Could you check a few things on this model? Use its own coordinates, in mm. Face numbers are marked on the shaded views. A direction names the side the tool comes from. Coordinates: 2 decimals unless noted, no trailing zeros. Write each loop counter-clockwise with the first axis right and the second up, starting at its lowest first coordinate (ties: lowest second). Pieces come first, ordered by that corner, then holes. Notation, with made-up numbers: M 77.5,-31 L 112.5,-31 A17 cw 112.5,-21 Z; hole C 11.5,28 d7. An arc over 180 degrees is marked long. Write item = value, one per line.
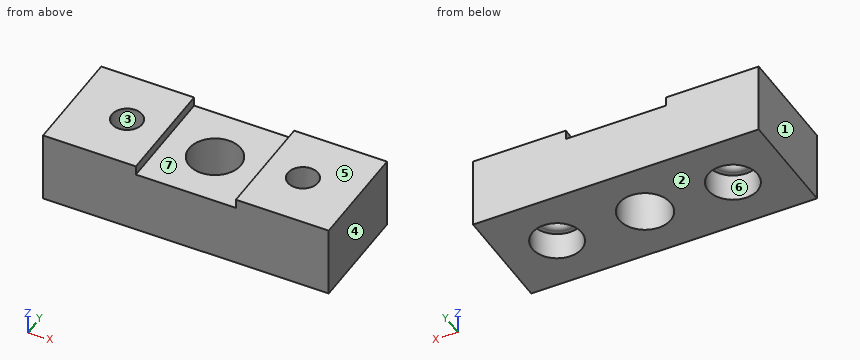
```python
from build123d import *

# Parameters (mm, degrees)
SKETCH_1_W          = 52
SKETCH_1_H          = 20
SKETCH_1_R          = 2.75
SKETCH_1_R_2        = 4.7
EXTRUDE_1_DEPTH     = 13
SKETCH_2_R          = 4.5
CUT_EXTRUDE_1_DEPTH = 5
SKETCH_3_W          = 18.2
SKETCH_3_H          = 20
CUT_EXTRUDE_2_DEPTH = 1.7
FILLET_1_R          = 1


with BuildPart() as part:
    # 草图1 → 凸台-拉伸1 (new body)
    with BuildSketch(Plane.XY):
        Rectangle(SKETCH_1_W, SKETCH_1_H)
        with Locations(Location((-16, 0, 0), (0, 0, 180))):
            Circle(SKETCH_1_R, mode=Mode.SUBTRACT)
        with Locations(Location((16, 0, 0), (0, 0, 180))):
            Circle(SKETCH_1_R, mode=Mode.SUBTRACT)
        with Locations(Location((0, 0, 0), (0, 0, 180))):
            Circle(SKETCH_1_R_2, mode=Mode.SUBTRACT)
    extrude(amount=EXTRUDE_1_DEPTH)

    # 草图2 → 切除-拉伸1 (cut)
    with BuildSketch(Plane(origin=(0, 0, 0), x_dir=(-1, 0, 0), z_dir=(0, 0, -1))):
        with Locations((-16, 0)):
            Circle(SKETCH_2_R)
        with Locations((16, 0)):
            Circle(SKETCH_2_R)
    extrude(amount=-CUT_EXTRUDE_1_DEPTH, mode=Mode.SUBTRACT)

    # 草图3 → 切除-拉伸2 (cut)
    with BuildSketch(Plane.XY.offset(13)):
        Rectangle(SKETCH_3_W, SKETCH_3_H)
    extrude(amount=-CUT_EXTRUDE_2_DEPTH, mode=Mode.SUBTRACT)

    # 圆角1
    fillet_1_edges = [part.edges().sort_by_distance(p)[0] for p in [
        (18.75, 0, 5),
        (-13.25, 0, 5),
    ]]
    fillet(fillet_1_edges, radius=FILLET_1_R)


solid = part.part
```
Item 1: If we mould it in two halves opening along X, with no side actions, what happens to the marked faces 1, 2, 3 and 4? For each: pulls with the +X half, pulls with the -X half, needs draft (parallel to the pull), parting line crosses it, or undercut.
Numbers:
face_1 = pulls with the -X half
face_2 = needs draft
face_3 = undercut
face_4 = pulls with the +X half
Item 2: Imagine slicing it at B-B (z = 8.25). Write out the boundary of the cut face in (x, y).
Numbers:
outline = M -26,-10 L 26,-10 L 26,10 L -26,10 Z; hole C -16,0 d5.5; hole C 0,0 d9.4; hole C 16,0 d5.5
Item 3: If I drill on line 1 along X through (y, z) = (0.25, 6.25); line 2 along Y through (x, z) = (0, 7.75); line 3 along X through (y, z) = (-4.25, 12), over which ranges is the centre line in solid material (lowest first)?
Numbers:
line_1 = -26 to -18.74, -13.26 to -4.69, 4.69 to 13.26, 18.74 to 26
line_2 = -10 to -4.7, 4.7 to 10
line_3 = -26 to -9.1, 9.1 to 26
Item 4: I'm going to push flat-ended pins straight in: P1, Ø7, axis at x = 16, y = 0, coming from the -Z side; P2, Ø9, axis at x = -4, y = 2.5, coming from the +Z side. Where does each tip first touch, or does it pass through?
Numbers:
P1 = 5.03
P2 = 11.3
Item 5: Imagine slicing it at D-D (y = 8.25). Write out the boundary of the cut face in (x, z), and give its area (3 significant figures).
Numbers:
outline = M -26,0 L 26,0 L 26,13 L 9.1,13 L 9.1,11.3 L -9.1,11.3 L -9.1,13 L -26,13 Z
area = 645 mm²
Item 6: For the marked faces 5, 6 and 7, which set-ups out of +Z, -Z, +X, -X, +Y, -Y let a thin tool reach every point of the face, with its end or its side?
Numbers:
face_5 = +Z, +X, -X, +Y, -Y
face_6 = -Z
face_7 = +Z, +Y, -Y
Item 7: Imagine slicing it at A-A (x = 0). Write out the boundary of the cut face in (y, z).
Numbers:
outline = M -10,0 L -4.7,0 L -4.7,11.3 L -10,11.3 Z; M 4.7,0 L 10,0 L 10,11.3 L 4.7,11.3 Z
Item 8: Imagine slicing it at C-C (y = 0). State how many separate pieces and enclosed holes the cut face has, and give its area (3 significant figures).
Numbers:
separate_pieces = 4
enclosed_holes = 0
area = 360 mm²
